Verification items for the finished model (mm, model axes). Face numbers are marked on the shaded views. A direction names the side the tool comes from. Round coordinates to 2 decimals unless told otherwise and drop trailing zeros. Order: outer loops, then holes, each group sorted by start corner. A loop starts at its lowest first (then second) coordinate and runs counter-clockwise, first axis right, second up. Notation, with made-up numbers: (70, 47) -> (78, 47) arc R17 ccw to (78, 57) -> close; hole circle Ø5 at (-25.75, 88). An arc over 180 degrees is marked (long way). Write item = value, one per line. Start each with the question number.
Autodesk Inventor part; units mm, degrees
ref_plane "YZ Plane" through (0, 0, 0) normal (1, 0, 0) x (0, 1, 0)
ref_plane "XZ Plane" through (0, 0, 0) normal (0, 1, 0) x (-1, 0, 0)
ref_plane "XY Plane" through (0, 0, 0) normal (0, 0, 1) x (1, 0, 0)
sketch "Sketch1" plane through (0, 0, 0) normal (0, 1, 0) x (-1, 0, 0)
  line L0 (0, 0) -> (-20.51, 0)
  line L1 (-20.51, 0) -> (-20.51, -10)
  line L2 (-20.51, -10) -> (0, -10)
  line L3 (0, -10) -> (0, 0)
  dimension "d0" = 20.51
  dimension "d1" = 10
extrude "Extrusion1" add sketch "Sketch1" along normal blind 6
sketch "Sketch3" plane through (20.51, 0, -10) normal (0, 0, -1) x (-1, 0, 0)
  line L0 (0, 0) -> (20.51, 0)
  circle A0 centre (10.255, 0) radius 4.75
  point P0 (15.005, 0)
  point P1 (5.505, 0)
  dimension "d4" = 9.5
extrude "Extrusion2" cut sketch "Sketch3" against normal through all contours A0 L0 picked at (11.657, 0.7358)
sketch "Sketch7" plane through (0, 6, 0) normal (0, 1, 0) x (1, 0, 0)
  line L0 (0, 0) -> (20.51, 0)
  line L1 (20.51, 10) -> (0, 10)
  line L2 (4.7, 0) -> (0, 0)
  line L3 (0, 0) -> (0, 10)
  line L4 (0, 10) -> (4.7, 10)
  line L5 (4.7, 10) -> (4.7, 0)
extrude "Extrusion3" cut sketch "Sketch7" against normal blind 3.6
sketch "Sketch8" plane through (0, 2.4, 0) normal (0, 1, 0) x (1, 0, 0)
  circle A0 centre (3, 5) radius 1.075
  point P0 (0, 0)
  dimension "d9" = 2.15
extrude "Extrusion4" cut sketch "Sketch8" against normal through all
chamfer "Chamfer1" distance 0.4 angle 45 1 edges at (1.925, 2.4, -5)
fillet "Fillet1" radius 2 2 edges at (4.7, 6, -5) (20.51, 6, -5)
properties part number "dg_clamp"
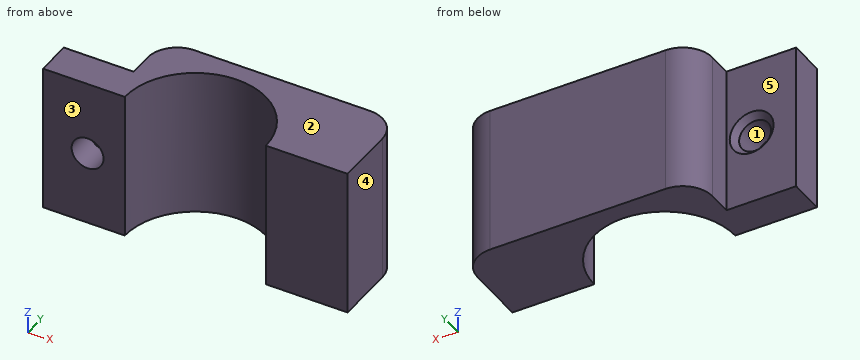
(1) Set-up check for the marked faces 4 and 5: record each of +Z, -Z, +X, -X, +Y, -Y from which the full face is reachable in a straight line by a thin tool's end or side.
(2) Cross-section at D-D (y = 5.6). Enter the section's corners in (x, z).
(3) Scan lines: line 1 along Z through (x, y) = (3, 1.65) (3 decimals); line 2 along X through (y, z) = (0.9, -5) (3 decimals); line 3 along X through (y, z) = (1.55, -5) (3 decimals). Record each from-to range of solid material in increasing order. Write a range as from..to.
(4) Cross-section at C-C (z = -6.75). Enter the section's corners in (x, y) (3 decimals).
(5) Cross-section at B-B (x = 3). Enter the section's corners in (y, z) (3 decimals).
(6) Draft check along Z on the marked faces 1, 2 and 3. Enter one of: +Z half, -Z half, draft (parallel to the pull), parting line (faces both ways), or undercut.
(7) Depth check by flat-ended pin: pin 1 (1.5 mm diameter, centred on y = 5, z = -4.5, fed in from +X); pin 2 (1.5 mm diameter, centred on x = 3.5, z = -5, fed in from +Y) (3 decimals); pin 3 (1.3 mm diameter, centred on x = 3, z = -5, fed in from +Y); pin 4 (4 mm diameter, centred on x = 1.5, z = -6.5, fed in from +Y). Enter the tip coordinate at first touch or a pass-through.
(8) Cross-section at A-A (z = -5). Enter the section's corners in (x, y) (3 decimals), and give its area (3 significant figures).
Outcome:
q1.face_4 = +Z, -Z, +X, +Y, -Y
q1.face_5 = +Z, -Z, -X, +Y
q2.outline = (5.5, -10) -> (19.71, -10) -> (19.71, 0) -> (5.5, 0) -> close
q3.line_1 = -10..-6.075, -3.925..0
q3.line_2 = 0..1.925, 4.075..5.591, 14.919..20.51
q3.line_3 = 0..1.925, 4.075..5.765, 14.745..20.51
q4.outline = (0, 0) -> (5.505, 0) arc R4.75 cw to (15.005, 0) -> (20.51, 0) -> (20.51, 4) arc R2 ccw to (18.51, 6) -> (6.7, 6) arc R2 ccw to (4.7, 4) -> (4.7, 2.4) -> (0, 2.4) -> close
q5.outline = (0, -10) -> (2.4, -10) -> (2.4, -6.475) -> (2, -6.075) -> (0, -6.075) -> close; (0, -3.925) -> (2, -3.925) -> (2.4, -3.525) -> (2.4, 0) -> (0, 0) -> close
q6.face_1 = undercut
q6.face_2 = +Z half
q6.face_3 = draft
q7.pin_1 = 20.49
q7.pin_2 = 2.175
q7.pin_3 = through
q7.pin_4 = 2.4
q8.outline = (0, 0) -> (1.925, 0) -> (1.925, 2) -> (1.525, 2.4) -> (0, 2.4) -> close; (4.075, 0) -> (5.505, 0) arc R4.75 cw to (15.005, 0) -> (20.51, 0) -> (20.51, 4) arc R2 ccw to (18.51, 6) -> (6.7, 6) arc R2 ccw to (4.7, 4) -> (4.7, 2.4) -> (4.475, 2.4) -> (4.075, 2) -> close
q8.area = 63.7 mm^2
